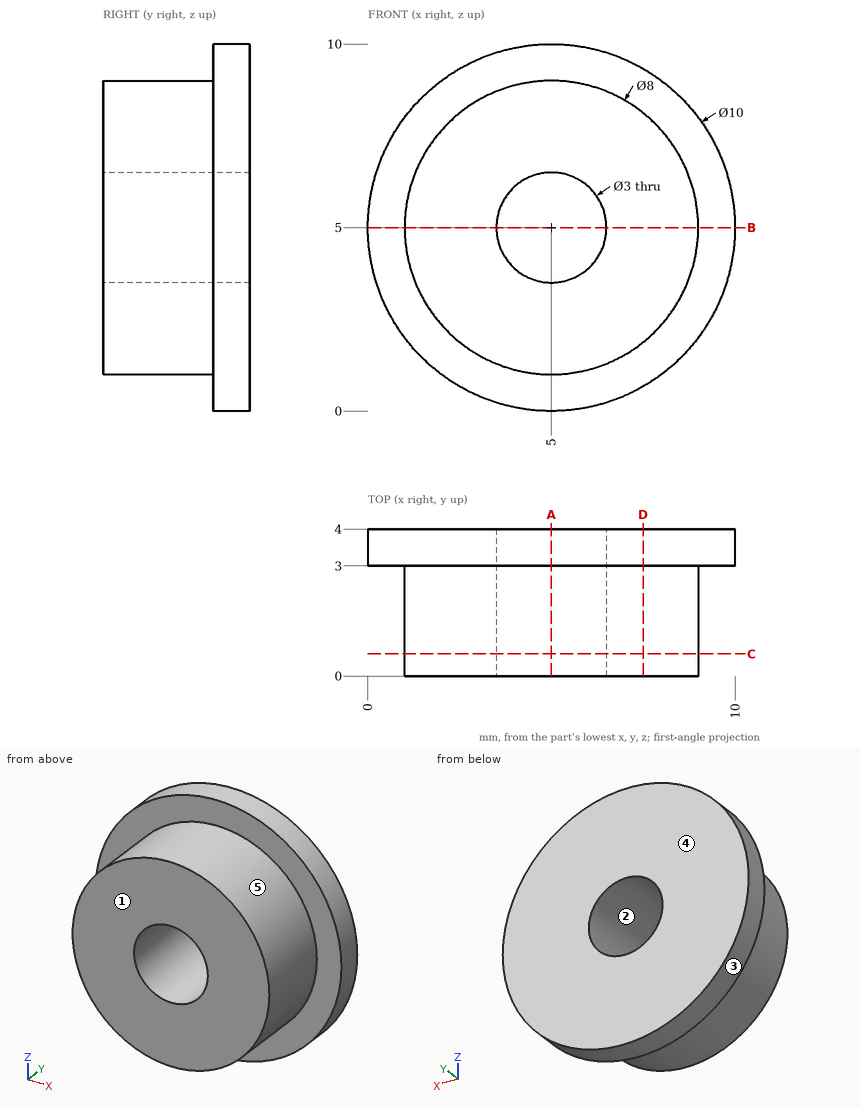
Drawing for the job (mm, zero at the part's lowest x, y, z). A direction names the side the tool comes from. Coordinates: 2 decimals unless noted, no trailing zeros. Order: outer loops, then holes, each group sorted by start corner. A loop starts at its lowest first (then second) coordinate and runs counter-clockwise, first axis right, second up. Notation, with made-up numbers: (-17, 6.25) -> (5, 6.25) arc R27 cw to (5, 35.25) -> close; hole circle Ø4 at (53.5, -36.5). An arc over 180 degrees is marked (long way). Return JSON: item names as keys, results as strings.
Item 1: 3-axis set-ups, long thin cutter, end or side, ignore diameter. For the marked faces 4 and 5: which of +Z, -Z, +X, -X, +Y, -Y reach the whole face in a straight line?
Model answer:
{"face 4": "+Z, -Z, +X, -X, +Y", "face 5": "-Y"}
Item 2: Slice it at B-B (z = 5). Write the cut outline in (x, y), then the cut area to 3 significant figures.
Model answer:
{"outline": "(0, 3) -> (1, 3) -> (1, 0) -> (3.5, 0) -> (3.5, 4) -> (0, 4) -> close; (6.5, 0) -> (9, 0) -> (9, 3) -> (10, 3) -> (10, 4) -> (6.5, 4) -> close", "area": "22.0 mm²"}
Item 3: Slice it at D-D (x = 7.5). Write the cut outline in (y, z), then the cut area to 3 significant figures.
Model answer:
{"outline": "(0, 1.88) -> (3, 1.88) -> (3, 0.67) -> (4, 0.67) -> (4, 9.33) -> (3, 9.33) -> (3, 8.12) -> (0, 8.12) -> close", "area": "27.4 mm²"}
Item 4: Slice it at A-A (x = 5). Write the cut outline in (y, z), then the cut area to 3 significant figures.
Model answer:
{"outline": "(0, 1) -> (3, 1) -> (3, 0) -> (4, 0) -> (4, 3.5) -> (0, 3.5) -> close; (0, 6.5) -> (4, 6.5) -> (4, 10) -> (3, 10) -> (3, 9) -> (0, 9) -> close", "area": "22.0 mm²"}
Item 5: Pin check, flat tip, straight feed: P1, Ø2, axis at x = 1.5, y = 2.5, coming from the -Z side. Stop position of the tip, or through.
Model answer:
{"P1": "stops at z = 0.75"}
Item 6: Wall check: line 1 along Z through (x, y) = (5, 2.5); line 2 along X through (y, z) = (1.8, 5.5). Give the ranges that are in metal, low to high. Write a range as from..to.
Model answer:
{"line 1": "z = 1..3.5, 6.5..9", "line 2": "x = 1.03..3.59, 6.41..8.97"}
Item 7: Slice it at C-C (y = 0.6). Write the cut outline in (x, z), then the cut area to 3 significant figures.
Model answer:
{"outline": "circle Ø8 at (5, 5); hole circle Ø3 at (5, 5)", "area": "43.2 mm²"}
Item 8: Mould opens along Z. For the marked faces 1, 2 and 3 say: pulls with the +Z half, pulls with the -Z half, needs draft (parallel to the pull), parting line crosses it, or undercut.
Model answer:
{"face 1": "needs draft", "face 2": "undercut", "face 3": "parting line crosses it"}
